CAD build for the part. Positions are in the model's coordinates, mm. Face numbers are marked on the shaded views. Round coordinates to 2 decimals unless told otherwise and drop trailing zeros. Order: outer loops, then holes, each group sorted by start corner. A loop starts at its lowest first (then second) coordinate and runs counter-clockwise, first axis right, second up. Notation, with made-up numbers: (44, -33.5) - (64, -33.5) arc R24 ccw to (64, -15.5) - close; hole circle Ø10 at (78, 45.25). An arc over 180 degrees is marked (long way). Write item = value, one per line.
from build123d import *

# Parameters (mm, degrees)
SKETCH2_R          = 2.38125
CUT_EXTRUDE1_DEPTH = 85.401041751
SKETCH5_R          = 10.16
SKETCH5_R_2        = 3.65125
CUT_EXTRUDE4_DEPTH = 50.8


with BuildPart() as part:
    # Sketch1 → Revolve1 (revolve)
    with BuildSketch(Plane.XY):
        with BuildLine():
            Line((0, 0), (0, -50.8))
            ThreePointArc((0, -50.8), (3.280951188, -68.760512242), (12.7, -84.401041651))
            Line((12.7, -84.401041651), (12.7, 0))
            Line((12.7, 0), (0, 0))
        make_face()
    revolve(axis=Axis((12.7, -84.401041651, 0), (0, 1, 0)))

    # Sketch2 → Cut-Extrude1 (cut, through all)
    with BuildSketch(Plane(origin=(0, 0, 0), x_dir=(1, 0, 0), z_dir=(0, 1, 0))):
        with Locations((12.7, 0)):
            Circle(SKETCH2_R)
    extrude(amount=-CUT_EXTRUDE1_DEPTH, mode=Mode.SUBTRACT)

    # Sketch5 → Cut-Extrude4 (cut)
    with BuildSketch(Plane(origin=(0, 0, 0), x_dir=(1, 0, 0), z_dir=(0, 1, 0))):
        with Locations((12.7, 0)):
            Circle(SKETCH5_R)
        with Locations((12.7, 0)):
            Circle(SKETCH5_R_2, mode=Mode.SUBTRACT)
    extrude(amount=-CUT_EXTRUDE4_DEPTH, mode=Mode.SUBTRACT)


solid = part.part
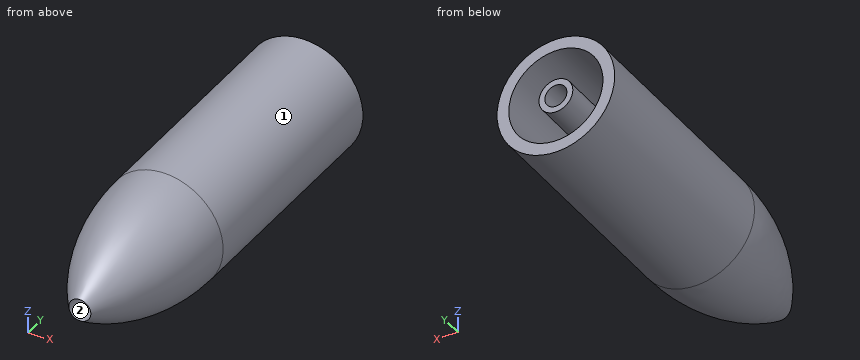
(1) Drop flat-ended pins along their axis: pin 1 (3 mm diameter, centred on x = 5.5, y = -34.5, fed in from +Z); pin 2 (3 mm diameter, centred on x = 22, y = -33.5, fed in from +Z); pin 3 (1.5 mm diameter, centred on y = -71.5, z = -7.5, fed in from +X). Give the stop position or say it passes through.
Solved:
pin_1 = 11.35
pin_2 = 10.02
pin_3 = 17.66
(2) Pull direction Z, two halves, no side cores. Call the marked faces 1 and 2: released by +Z, released by -Z, zero draft, split by the parting line, or undercut.
Solved:
face_1 = split by the parting line
face_2 = undercut
(3) Probe line 1 along Z through (x, y) = (12.7, -29); line 2 along Z through (x, y) = (11.5, -31.5); line 3 along X through (y, z) = (-37.5, -8.75). List the from-to ranges inside material, lowest first.
Solved:
line_1 = -12.7 to -10.16, -3.65 to -2.38, 2.38 to 3.65, 10.16 to 12.7
line_2 = -12.64 to -10.09, -3.45 to -2.06, 2.06 to 3.45, 10.09 to 12.64
line_3 = 3.5 to 7.54, 17.86 to 21.9
(4) Band-saw the part on A-A on y = -28.5. List the corners of the cut face in (x, z), plus the area to 3 significant figures.
Solved:
outline = circle Ø25.4 at (12.7, 0); circle Ø7.3 at (12.7, 0); hole circle Ø20.32 at (12.7, 0); hole circle Ø4.76 at (12.7, 0)
area = 206 mm²
